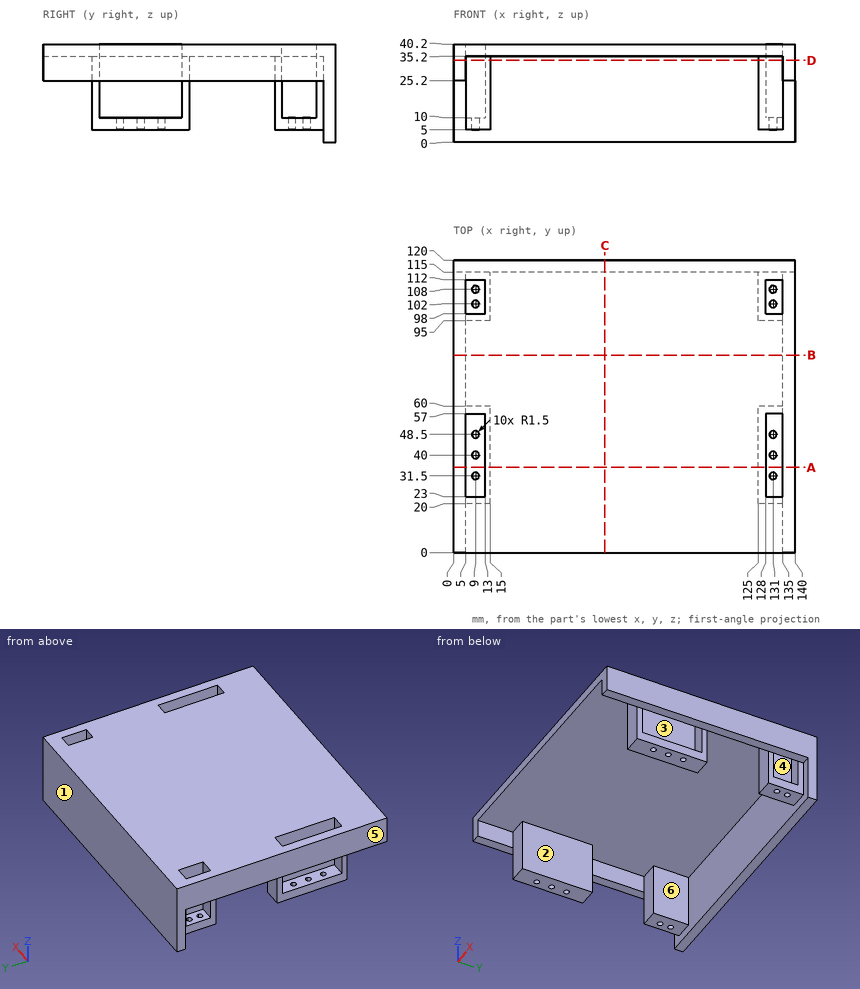
Input: dimensioned drawing with shaded views. Units: mm. Origin: part minimum x, y, z. A direction names the side the tool comes from. Round coordinates to 2 decimals unless told otherwise and drop trailing zeros. Loops run counter-clockwise (first coordinate to the right, second up) from the corner with the lowest first, then second, coordinate; pieces in that order, holes last. Notation, with made-up numbers: M -7,-3 L 31,-3 A19 ccw 31,15 Z; hole C 75.25,-30.5 d5. An arc over 180 degrees is marked long. Return JSON: item names as keys, results as strings. Group by question number.
1. Mould query, pull axis Y, two halves, no side actions, for the marked faces 1, 2 and 3. Classes: released by +Y, released by -Y, zero draft, split by the parting line, or undercut.
2. Reachability of the marked faces 4, 5 and 6 from +Z, -Z, +X, -X, +Y, -Y: full face, straight path, thin tool, end or side. Return the list, or none.
3. Section query B-B on y = 81. Output: boundary loops of the cut face in (x, z), and give its area (3 significant figures).
4. Section query C-C on x = 62. Output: boundary loops of the cut face in (y, z).
5. Material intervals for line 1 along X through (y, z) = (52.5, 15); line 2 along X through (y, z) = (19.5, 30); line 3 along Z through (x, y) = (98, 11.5), sorted ascending. Write a range as from..to.
6. Pin query (flat end, axial travel): pin 1 (16 mm diameter, centred on y = 104, z = 10, fed in from +X); pin 2 (3 mm diameter, centred on x = 131, z = 24, fed in from -Y); pin 3 (5 mm diameter, centred on x = 89.5, z = 25, fed in from -Y). Return the tip coordinate at first contact, or that it passes through.
7. Section query D-D on z = 33.5. State how many separate pieces and enclosed holes the cut face has, and give its area (3 significant figures).
8. Section query A-A on y = 35. Output: boundary loops of the cut face in (x, z).
Checks:
{
 "1": {"face 1": "released by +Y", "face 2": "zero draft", "face 3": "undercut"},
 "2": {"face 4": "+Z", "face 5": "+Z, -Z, -X, +Y, -Y", "face 6": "-Z, -Y"},
 "3": {"outline": "M 0,25.2 L 5,25.2 L 5,35.2 L 135,35.2 L 135,25.2 L 140,25.2 L 140,40.2 L 0,40.2 Z", "area": "800 mm²"},
 "4": {"outline": "M 0,35.2 L 115,35.2 L 115,0 L 120,0 L 120,40.2 L 0,40.2 Z"},
 "5": {"line 1": "x = 13..15, 125..128", "line 2": "x = 0..5, 135..140", "line 3": "z = 35.2..40.2"},
 "6": {"pin 1": "stops at x = 135", "pin 2": "stops at y = 20", "pin 3": "stops at y = 115"},
 "7": {"separate pieces": "1", "enclosed holes": "4", "area": "2,330 mm²"},
 "8": {"outline": "M 0,25.2 L 5,25.2 L 5,40.2 L 0,40.2 Z; M 5,5 L 15,5 L 15,35.2 L 125,35.2 L 125,5 L 135,5 L 135,10 L 128,10 L 128,40.2 L 13,40.2 L 13,10 L 5,10 Z; M 135,25.2 L 140,25.2 L 140,40.2 L 135,40.2 Z"}
}
